The listing builds one solid part. Answer for the finished solid, in the listing's coordinates (mm). A direction names the side the tool comes from. Coordinates: 2 decimals unless noted, no trailing zeros. Order: outer loops, then holes, each group sorted by start corner. A loop starts at its lowest first (then second) coordinate and runs counter-clockwise, first axis right, second up. Notation, with made-up numbers: (13.25, -5) -> (40.25, -5) arc R19 ccw to (40.25, 5) -> close; hole circle Ø3 at (-22, 19). An arc over 180 degrees is marked (long way). Write each question's results on one line, items separated by ' | '. Start each with the question number.
(1) Determine the mould class of faces 1 (the face through (64.944, -3.252, 215.535)), 2 (the face through (43, -4.134, 101)), 3 (the face through (43.65, -1.845, 225.734)) for opening direction Z: +Z half, -Z half, draft (parallel to the pull), parting line (faces both ways), or undercut.
(2) Straight lines are drawn through the part: L1, parallel to Y at x = 22, z = 11; L2, parallel to X at y = -0.5, z = 28.5; L3, parallel to Z at x = 84, y = -1.5. For each, find the intervals that lie inside material, in ascending order.
(3) The part is cut by section A-A, the plane z = 200.5. Give the vertices of the cut face in (x, y).
(4) The part is cut by section B-B, the plane z = 5.5. Give the vertices of the cut face in (x, y).
(5) A tool of negligible diameter and unlimited length cuts with its end or side. For faces 4 (the face through (43.65, -0.566, -26.565)), 5 (the face through (43, -3.134, 98)), 6 (the face through (2, 0, 98)), from which of +Z, -Z, +X, -X, +Y, -Y can it reach the whole face along a straight path? Write none if from no direction.
(6) Given pin 1 (3 mm diameter, centred on y = 0, z = -35, fed in from -X); pin 2 (0.8 mm diameter, centred on x = 58, y = -1.5, fed in from +Z); pin 3 (0.9 mm diameter, centred on y = -3.5, z = 207, fed in from -X), each flat-ended and moving along its own axis, determine where each tip first touches the part or whether it passes through.
```python
from build123d import *

# Parameters (mm, degrees)
BOSS_EXTRUDE1_DEPTH      = 197
CUT_EXTRUDE3_DEPTH       = 216.79851714
CUT_EXTRUDE3_DEPTH_BACK  = 216.79851714
BOSS_EXTRUDE2_DEPTH      = 88
CUT_EXTRUDE4_DEPTH       = 216.82432282
CUT_EXTRUDE4_DEPTH_BACK  = 216.82432282
BOSS_EXTRUDE3_DEPTH      = 88
CUT_EXTRUDE_Q_DEPTH      = 257.591354983
CUT_EXTRUDE_Q_DEPTH_BACK = 257.591354983
SKETCH11_R               = 1.5
SKETCH11_R_2             = 1
CUT_EXTRUDE5_DEPTH       = 10
SKETCH12_R               = 1.5
SKETCH12_R_2             = 1
CUT_EXTRUDE6_DEPTH       = 10
SKETCH14_R               = 1.5
SKETCH14_R_2             = 1
CUT_EXTRUDE7_DEPTH       = 10
SKETCH16_R               = 1.5
CUT_EXTRUDE8_DEPTH       = 10


with BuildPart() as part:
    # Sketch1 → Boss-Extrude1 (new body)
    with BuildSketch(Plane.XY):
        Polygon((0, 0), (7.160254038, -4.133974596), (80.839745962, -4.133974596), (88, 0), (87.5, 0.866025404), (80.57179677, -3.133974596), (7.42820323, -3.133974596), (0.5, 0.866025404), align=None)
    extrude(amount=BOSS_EXTRUDE1_DEPTH)

    # Sketch3 → Cut-Extrude3 (cut, two sides: drawn at the far end of the back side and taken through both)
    with BuildSketch(Plane(origin=(0, -3.133974596, 0), x_dir=(1, 0, 0), z_dir=(0, 1, 0)).offset(-CUT_EXTRUDE3_DEPTH_BACK)):
        Polygon((0, 0), (0, -17), (7.42820323, -11.738356045), (7.42820323, 0), align=None)
        Polygon((7.42820323, 0), (7.42820323, -11.738356045), (24, 0), align=None)
        Polygon((80.57179677, 0), (64, 0), (80.57179677, -11.738356045), align=None)
        Polygon((80.57179677, 0), (80.57179677, -11.738356045), (88, -17), (88, 0), align=None)
        Polygon((7.42820323, -186.037245166), (0, -179), (0, -197), (7.42820323, -197), align=None)
        Polygon((19, -197), (7.42820323, -186.037245166), (7.42820323, -197), align=None)
        Polygon((80.57179677, -186.037245166), (69, -197), (80.57179677, -197), align=None)
        Polygon((88, -179), (80.57179677, -186.037245166), (80.57179677, -197), (88, -197), align=None)
    extrude(amount=CUT_EXTRUDE3_DEPTH + CUT_EXTRUDE3_DEPTH_BACK, mode=Mode.SUBTRACT)

    # Sketch5 → Boss-Extrude2 (add)
    with BuildSketch(Plane(origin=(0, 0, 0), x_dir=(0, 0, -1), z_dir=(1, 0, 0))):
        Polygon((0, -3.133974596), (12, -3.133974596), (41.54423259, 2.075470734), (41.717880768, 1.090662981), (12.087488664, -4.133974596), (0, -4.133974596), align=None)
    extrude(amount=BOSS_EXTRUDE2_DEPTH)

    # Sketch6 → Cut-Extrude4 (cut, two sides: drawn at the far end of the back side and taken through both)
    with BuildSketch(Plane(origin=(0, -3.133974596, 0), x_dir=(1, 0, 0), z_dir=(0, 1, 0)).offset(-CUT_EXTRUDE4_DEPTH_BACK)):
        with BuildLine():
            Line((24, 0), (30, 0))
            Line((30, 0), (30, 3))
            Line((30, 3), (27.5, 3))
            Line((27.5, 3), (27.5, 12.087488664))
            ThreePointArc((27.5, 12.087488664), (26.488631596, 14.746074976), (23.96595941, 16.060256191))
            Line((23.96595941, 16.060256191), (19, 16.642705453))
            Line((19, 16.642705453), (19, 21.642705453))
            Line((19, 21.642705453), (22.366709334, 22.599401987))
            ThreePointArc((22.366709334, 22.599401987), (24.989583103, 24.39514756), (26, 27.40898675))
            Line((26, 27.40898675), (26, 41.717880768))
            Line((26, 41.717880768), (62, 41.717880768))
            Line((62, 41.717880768), (62, 27.40898675))
            ThreePointArc((62, 27.40898675), (63.010416897, 24.39514756), (65.633290666, 22.599401987))
            Line((65.633290666, 22.599401987), (69, 21.642705453))
            Line((69, 21.642705453), (69, 16.642705453))
            Line((69, 16.642705453), (64.03404059, 16.060256191))
            ThreePointArc((64.03404059, 16.060256191), (61.511368404, 14.746074976), (60.5, 12.087488664))
            Line((60.5, 12.087488664), (60.5, 3))
            Line((60.5, 3), (58, 3))
            Line((58, 3), (58, 0))
            Line((58, 0), (64, 0))
            Line((64, 0), (89.345545356, 0))
            Line((89.345545356, 0), (89.345545356, 57.606108668))
            Line((89.345545356, 57.606108668), (-1.345545356, 57.606108668))
            Line((-1.345545356, 57.606108668), (-1.345545356, 0))
            Line((-1.345545356, 0), (24, 0))
        make_face()
    extrude(amount=CUT_EXTRUDE4_DEPTH + CUT_EXTRUDE4_DEPTH_BACK, mode=Mode.SUBTRACT)

    # Sketch8 → Boss-Extrude3 (add)
    with BuildSketch(Plane(origin=(0, 0, 0), x_dir=(0, 0, -1), z_dir=(1, 0, 0))):
        Polygon((-197, -3.133974596), (-211, -3.133974596), (-240.885840943, -0.519302314), (-240.972996686, -1.515497012), (-211.043660943, -4.133974596), (-197, -4.133974596), align=None)
    extrude(amount=BOSS_EXTRUDE3_DEPTH)

    # Sketch9 → Cut-Extrude q (cut, two sides: drawn at the far end of the back side and taken through both)
    with BuildSketch(Plane(origin=(0, -3.133974596, 0), x_dir=(1, 0, 0), z_dir=(0, 1, 0)).offset(-CUT_EXTRUDE_Q_DEPTH_BACK)):
        with BuildLine():
            Line((29, -221.608495283), (29, -236.972996686))
            Line((29, -236.972996686), (31.84982933, -236.972996686))
            Line((31.84982933, -236.972996686), (31.84982933, -240.972996686))
            Line((31.84982933, -240.972996686), (31.84982933, -252.017077063))
            Line((31.84982933, -252.017077063), (0, -252.017077063))
            Line((0, -252.017077063), (0, -240.885840943))
            Line((0, -240.885840943), (0, -211))
            Line((0, -211), (0, -197))
            Line((0, -197), (19, -197))
            ThreePointArc((19, -197), (22.5, -200.5), (19, -204))
            Line((19, -204), (19, -213))
            Line((19, -213), (27, -218))
            ThreePointArc((27, -218), (28.466564953, -219.545655117), (29, -221.608495283))
        make_face()
        with BuildLine():
            Line((88, -211), (88, -240.885840943))
            Line((88, -240.885840943), (88, -252.017077063))
            Line((88, -252.017077063), (56.15017067, -252.017077063))
            Line((56.15017067, -252.017077063), (56.15017067, -240.972996686))
            Line((56.15017067, -240.972996686), (56.15017067, -236.972996686))
            Line((56.15017067, -236.972996686), (59, -236.972996686))
            Line((59, -236.972996686), (59, -221.608495283))
            ThreePointArc((59, -221.608495283), (59.533435047, -219.545655117), (61, -218))
            Line((61, -218), (69, -213))
            Line((69, -213), (69, -204))
            ThreePointArc((69, -204), (65.5, -200.5), (69, -197))
            Line((69, -197), (88, -197))
            Line((88, -197), (88, -211))
        make_face()
    extrude(amount=CUT_EXTRUDE_Q_DEPTH + CUT_EXTRUDE_Q_DEPTH_BACK, mode=Mode.SUBTRACT)

    # Sketch11 → Cut-Extrude5 (cut)
    with BuildSketch(Plane(origin=(0, -22.42624598, 1.962042289), x_dir=(1, 0, 0), z_dir=(0, -0.9961946980917457, 0.08715574274765849))):
        with Locations(Location((39.5, 232.923937414, 0), (0, 0, 270))):
            Circle(SKETCH11_R)
        with Locations(Location((31, 206.923937414, 0), (0, 0, 90))):
            Circle(SKETCH11_R)
        with Locations(Location((40.5, 206.423937414, 0), (0, 0, 90))):
            Circle(SKETCH11_R_2)
        with Locations(Location((47.5, 206.423937414, 0), (0, 0, 90))):
            Circle(SKETCH11_R_2)
        with Locations(Location((57, 206.923937414, 0), (0, 0, 90))):
            Circle(SKETCH11_R)
        with Locations(Location((48.5, 232.923937414, 0), (0, 0, 270))):
            Circle(SKETCH11_R)
    extrude(amount=-CUT_EXTRUDE5_DEPTH, mode=Mode.SUBTRACT)

    # Sketch12 → Cut-Extrude6 (cut)
    with BuildSketch(Plane(origin=(0, 0, 0), x_dir=(0.866025403784438, -0.5000000000000012, 0), z_dir=(-0.5000000000000011, -0.8660254037844379, 0))):
        with Locations((4.133974596, 177.391699281)):
            Circle(SKETCH12_R)
        with Locations((4.133974596, 98.427887988)):
            Circle(SKETCH12_R)
        with Locations((4.133974596, 20.964076695)):
            Circle(SKETCH12_R)
        with Locations(Location((8.267949192, 20.464076695, 0), (0, 0, 270))):
            Circle(SKETCH12_R_2)
    cut_extrude6 = extrude(amount=-CUT_EXTRUDE6_DEPTH, mode=Mode.SUBTRACT)

    # Mirror1: Cut-Extrude6 across plane
    add(cut_extrude6.mirror(Plane(origin=(44, 0, 0), x_dir=(0, 0, 1), z_dir=(1, 0, 0))), mode=Mode.SUBTRACT)

    # Sketch14 → Cut-Extrude7 (cut)
    with BuildSketch(Plane.XZ.offset(4.133974596)):
        with Locations((30.5, 184)):
            Circle(SKETCH14_R)
        with Locations((22.5, 15)):
            Circle(SKETCH14_R)
        with Locations((44, 177)):
            Circle(SKETCH14_R)
        with Locations(Location((65.5, 15, 0), (0, 0, 270))):
            Circle(SKETCH14_R)
        with Locations(Location((57.5, 184, 0), (0, 0, 270))):
            Circle(SKETCH14_R)
        with Locations((71, 177)):
            Circle(SKETCH14_R)
        with Locations((9, 137)):
            Circle(SKETCH14_R)
        with Locations((32, 105)):
            Circle(SKETCH14_R)
        with Locations((32, 137)):
            Circle(SKETCH14_R)
        with Locations((9, 105)):
            Circle(SKETCH14_R)
        with Locations((13, 28.5)):
            Circle(SKETCH14_R)
        with Locations((35.5, 28.5)):
            Circle(SKETCH14_R)
        with Locations((56, 28.5)):
            Circle(SKETCH14_R)
        with Locations((59.5, 28.5)):
            Circle(SKETCH14_R_2)
        with Locations((56, 75)):
            Circle(SKETCH14_R)
        with Locations((56, 60)):
            Circle(SKETCH14_R)
        with Locations((55.5, -10.087488664)):
            Circle(SKETCH14_R)
        with Locations((32.5, -10.087488664)):
            Circle(SKETCH14_R)
        with Locations((46.5, -9.587488664)):
            Circle(SKETCH14_R_2)
        with Locations((41.5, -9.587488664)):
            Circle(SKETCH14_R_2)
        with Locations((59.5, 60)):
            Circle(SKETCH14_R_2)
    extrude(amount=-CUT_EXTRUDE7_DEPTH, mode=Mode.SUBTRACT)

    # Sketch16 → Cut-Extrude8 (cut)
    with BuildSketch(Plane(origin=(0, -6.076402312, -1.071433673), x_dir=(1, 0, 0), z_dir=(0, -0.9848077530122079, -0.17364817766693125))):
        with Locations(Location((38, -37.273484059, 0), (0, 0, 270))):
            Circle(SKETCH16_R)
        with Locations(Location((50, -37.273484059, 0), (0, 0, 270))):
            Circle(SKETCH16_R)
    extrude(amount=-CUT_EXTRUDE8_DEPTH, mode=Mode.SUBTRACT)


solid = part.part
```
Established:
1) face 1: +Z half | face 2: draft | face 3: undercut
2) L1: y = -4.13 to -3.13 | L2: x = 0.87 to 2.87, 85.13 to 87.13 | L3: z = 14.17 to 19.47, 22.46 to 96.93, 99.93 to 175.89, 178.89 to 182.79
3) outline: (22.5, -4.13) -> (65.5, -4.13) -> (65.5, -3.13) -> (22.5, -3.13) -> close
4) outline: (16.24, -4.13) -> (71.76, -4.13) -> (71.76, -3.13) -> (16.24, -3.13) -> close
5) face 4: +X, -X, +Y | face 5: +Y | face 6: +Z, -Z, +Y
6) pin 1: stops at x = 26 | pin 2: stops at z = 236.97 | pin 3: stops at x = 19
